Can you work these out from the model? Positions are in its coordinate system, mm. A direction names the side the tool comes from. Round coordinates to 2 decimals unless told otherwise and drop trailing zeros. Loops run counter-clockwise (first coordinate to the right, second up) from the corner with the lowest first, then second, coordinate; pieces in that order, holes last. Notation, with made-up numbers: (66.5, -31.5) -> (98.5, -31.5) arc R20 ccw to (98.5, 4.5) -> close; hole circle Ø2 at (17, -24.75). An arc over 180 degrees is marked (long way). Write each question's results on one line, items separated by ' | '.
from build123d import *

# Parameters (mm, degrees)
F0_R     = 63.5
F1_DEPTH = 12.7
F3_DEPTH = 63.5
F4_W     = 25.4
F4_H     = 50.8
F5_DEPTH = 50.8
F7_DEPTH = 127
F8_R     = 25.39999
F9_R     = 3.81


# Not quite as in the source:
# - a fillet or chamfer is up to 0.001 mm smaller than in the source, because OpenCascade refuses the exact size


with BuildPart() as f1:
    # F0 (on Top) → F1 (new body)
    with BuildSketch(Plane.XY):
        Circle(F0_R)
        with BuildLine():
            ThreePointArc((6.3279129766, -37.5708333333), (6.3444758413, -37.835186293), (6.35, -38.1))
            ThreePointArc((6.35, -38.1), (-0.264813707, -44.4444758413), (-6.3279129766, -37.5708333333))
            ThreePointArc((-6.3279129766, -37.5708333333), (0, -31.75), (6.3279129766, -37.5708333333))
        make_face(mode=Mode.SUBTRACT)
        with BuildLine():
            ThreePointArc((-37.5708333333, 6.3279129766), (-33.4265265416, 4.2989703225), (-31.75, 0))
            ThreePointArc((-31.75, 0), (-33.4265265416, -4.2989703225), (-37.5708333333, -6.3279129766))
            ThreePointArc((-37.5708333333, -6.3279129766), (-44.45, 0), (-37.5708333333, 6.3279129766))
        make_face(mode=Mode.SUBTRACT)
        with BuildLine():
            ThreePointArc((37.5708333333, -6.3279129766), (33.4265265416, -4.2989703225), (31.75, 0))
            ThreePointArc((31.75, 0), (33.4265265416, 4.2989703225), (37.5708333333, 6.3279129766))
            ThreePointArc((37.5708333333, 6.3279129766), (42.3989703225, 4.6734734584), (44.45, 0))
            ThreePointArc((44.45, 0), (42.3989703225, -4.6734734584), (37.5708333333, -6.3279129766))
        make_face(mode=Mode.SUBTRACT)
        with BuildLine():
            ThreePointArc((6.35, 38.1), (6.3444758413, 37.835186293), (6.3279129766, 37.5708333333))
            ThreePointArc((6.3279129766, 37.5708333333), (4.2989703225, 33.4265265416), (0, 31.75))
            ThreePointArc((0, 31.75), (-4.2989703225, 33.4265265416), (-6.3279129766, 37.5708333333))
            ThreePointArc((-6.3279129766, 37.5708333333), (-0.264813707, 44.4444758413), (6.35, 38.1))
        make_face(mode=Mode.SUBTRACT)
    extrude(amount=F1_DEPTH)

    # F2 (on face) → F3 (join)
    with BuildSketch(Plane.XY.offset(12.7)):
        Polygon((25.4, 25.4), (0, 25.4), (-25.4, 25.4), (-25.4, -25.4), (25.4, -25.4), align=None)
    extrude(amount=F3_DEPTH)

    # F4 (on face) → F5 (cut)
    with BuildSketch(Plane.XZ.offset(25.4)):
        with Locations((0, 50.8)):
            Rectangle(F4_W, F4_H)
    extrude(amount=-F5_DEPTH, mode=Mode.SUBTRACT)

    # F6 (on face) → F7 (cut)
    with BuildSketch(Plane.YZ.offset(25.4)):
        with BuildLine():
            ThreePointArc((9.525, 50.8), (6.7351920908, 57.5351920908), (0, 60.325))
            Line((0, 60.325), (0, 50.8))
            Line((0, 50.8), (0, 41.275))
            ThreePointArc((0, 41.275), (6.7351920908, 44.0648079092), (9.525, 50.8))
        make_face()
        with BuildLine():
            Line((0, 50.8), (0, 60.325))
            ThreePointArc((0, 60.325), (-9.525, 50.8), (0, 41.275))
            Line((0, 41.275), (0, 50.8))
        make_face()
    extrude(amount=-F7_DEPTH, mode=Mode.SUBTRACT)

    # F8 (radius 25.4 in the source; OpenCascade refuses exactly that, so slightly less here)
    f8_edges = [f1.edges().sort_by_distance(p)[0] for p in [
        (19.05, -25.4, 76.2),
        (19.05, 25.4, 76.2),
        (-19.05, -25.4, 76.2),
        (-19.05, 25.4, 76.2),
    ]]
    fillet(f8_edges, radius=F8_R)

    # F9
    f9_edges = [f1.edges().sort_by_distance(p)[0] for p in [
        (-63.5, 0, 12.7),
        (25.4, 0, 12.7),
        (0, -25.4, 12.7),
        (0, 25.4, 12.7),
        (-25.4, 0, 12.7),
    ]]
    fillet(f9_edges, radius=F9_R)


solid = f1.part
1. Please list where these lines run through material, in increasing order: line 1 (X direction, y = 18, z = 62); line 2 (Y direction, x = -20, z = 50.8) (3 decimals); line 3 (Z direction, x = 15, y = 0) (3 decimals). Write a range as from..to.
Final values:
line 1: -25.4..-12.7, 12.7..25.4 | line 2: -25.4..-9.525, 9.525..25.4 | line 3: 0..41.275, 60.325..76.2
2. If we section it at C-C (z = 6.5): List the corners of the cut face in (x, y) for me, then the cut area to 3 significant figures.
Final values:
outline: circle Ø127 at (0, 0); hole circle Ø12.7 at (-38.1, 0); hole circle Ø12.7 at (0, -38.1); hole circle Ø12.7 at (0, 38.1); hole circle Ø12.7 at (38.1, 0) | area: 12,200 mm2
3. If we section it at B-B (z = 56): List the corners of the cut face in (x, y) for me, then the cut area to 3 significant figures.
Final values:
outline: (-25.4, -24.86) -> (-12.7, -24.86) -> (-12.7, -7.98) -> (-25.4, -7.98) -> close; (-25.4, 7.98) -> (-12.7, 7.98) -> (-12.7, 24.86) -> (-25.4, 24.86) -> close; (12.7, -24.86) -> (25.4, -24.86) -> (25.4, -7.98) -> (12.7, -7.98) -> close; (12.7, 7.98) -> (25.4, 7.98) -> (25.4, 24.86) -> (12.7, 24.86) -> close | area: 858 mm2
4. If we section it at A-A (z = 36.5): List the corners of the cut face in (x, y) for me, then the cut area to 3 significant figures.
Final values:
outline: (-25.4, -25.4) -> (-12.7, -25.4) -> (-12.7, 25.4) -> (-25.4, 25.4) -> close; (12.7, -25.4) -> (25.4, -25.4) -> (25.4, 25.4) -> (12.7, 25.4) -> close | area: 1,290 mm2
5. On a 3-axis mill with a long thin cutter (end or side, diameter ignored), from which of +Z, -Z, +X, -X, +Y, -Y can I reach the whole of each face in a straight line? I mean faces 5 (the face through (0, 0, 25.4)), 6 (the face through (25.4, 0, 39)), 7 (the face through (0, -25.4, 22)). Say none if no direction works.
Final values:
face 5: +Z, +Y, -Y | face 6: +Z, +X, +Y, -Y | face 7: +Z, +X, -X, -Y
6. Will these pins go through, and if not, where does the flat tip stop? pin 1 (4 mm diameter, centred on y = -5, z = 18.5, fed in from -X); pin 2 (25 mm diameter, centred on y = 0, z = 50.8, fed in from +X); pin 3 (20.5 mm diameter, centred on x = 2, y = 8, fed in from +Z).
Final values:
pin 1: x = -25.4 | pin 2: x = 25.4 | pin 3: z = 25.4
7. We'd pull the mould along Y, two halves only. Please class faces 1 (the face through (-19.14, 18.16, 68.56)), 2 (the face through (-18.96, -2.06, 41.5)), 3 (the face through (26.546, 0.409, 13.786)), 4 (the face through (19.14, -2.06, 41.5)): pulls with the +Y half, pulls with the -Y half, needs draft (parallel to the pull), parting line crosses it, or undercut.
Final values:
face 1: pulls with the +Y half | face 2: undercut | face 3: needs draft | face 4: undercut
